from build123d import *

# Parameters (mm, degrees)
F0_R     = 25.118171
F0_R_2   = 20.499511
F1_DEPTH = 3
F0_R_3   = 15.56051
F2_DEPTH = 6
F0_R_4   = 10.077098
F3_DEPTH = 9
F0_R_5   = 4.284834
F4_DEPTH = 12
F0_R_6   = 1.253912
F5_DEPTH = 15
F6_DEPTH = 15
F7_DEPTH = 15


with BuildPart() as f1:
    # F0 (on Front) → F1 (new body)
    with BuildSketch(Plane.XZ):
        Circle(F0_R)
        Circle(F0_R_2, mode=Mode.SUBTRACT)
    extrude(amount=F1_DEPTH)

    # F0 (on Front) → F2 (join)
    with BuildSketch(Plane.XZ):
        Circle(F0_R_2)
        Circle(F0_R_3, mode=Mode.SUBTRACT)
    extrude(amount=F2_DEPTH)

    # F0 (on Front) → F3 (join)
    with BuildSketch(Plane.XZ):
        Circle(F0_R_3)
        Circle(F0_R_4, mode=Mode.SUBTRACT)
    extrude(amount=F3_DEPTH)

    # F0 (on Front) → F4 (join)
    with BuildSketch(Plane.XZ):
        Circle(F0_R_4)
        Circle(F0_R_5, mode=Mode.SUBTRACT)
    extrude(amount=F4_DEPTH)

    # F0 (on Front) → F5 (join)
    with BuildSketch(Plane.XZ):
        Circle(F0_R_5)
        Circle(F0_R_6, mode=Mode.SUBTRACT)
    extrude(amount=F5_DEPTH)

    # F0 (on Front) → F6 (join)
    with BuildSketch(Plane.XZ):
        Circle(F0_R_6)
    extrude(amount=F6_DEPTH)

    # F0 (on Front) → F7 (join)
    with BuildSketch(Plane.XZ):
        Circle(F0_R_6)
    extrude(amount=-F7_DEPTH)


solid = f1.part
For this review, take the finished solid that the model builds, in its own axes (mm). A direction names the side the tool comes from. Round coordinates to 2 decimals unless told otherwise and drop trailing zeros. Write each loop counter-clockwise with the first axis right and the second up, starting at its lowest first coordinate (ties: lowest second). Pieces come first, ordered by that corner, then holes. Notation, with made-up numbers: (-31, -8.75) -> (19, -8.75) arc R14 cw to (19, -4.75) -> close; hole circle Ø2 at (89.5, 66.25). An arc over 180 degrees is marked (long way). Use CSV: the item, a comma, the result in double quotes.
(1) Consider section A-A, the plane x = 0. Give the boundary of the cut face in (y, z).
Computed values:
outline,"(-15, -4.28) -> (-12, -4.28) -> (-12, -10.08) -> (-9, -10.08) -> (-9, -15.56) -> (-6, -15.56) -> (-6, -20.5) -> (-3, -20.5) -> (-3, -25.12) -> (0, -25.12) -> (0, -1.25) -> (15, -1.25) -> (15, 1.25) -> (0, 1.25) -> (0, 25.12) -> (-3, 25.12) -> (-3, 20.5) -> (-6, 20.5) -> (-6, 15.56) -> (-9, 15.56) -> (-9, 10.08) -> (-12, 10.08) -> (-12, 4.28) -> (-15, 4.28) -> close"
(2) Draft analysis for pull direction Z (two halves, no side actions). For faces 1 (the face through (-4.444, -4.479, -20.012)), 2 (the face through (3, -9, -10)), state which applies: +Z half, -Z half, draft (parallel to the pull), parting line (faces both ways), or undercut.
Computed values:
face 1,"parting line"
face 2,"draft"
(3) To check wall thickness, follow L1, parallel to Y at x = 7.5, z = -4.5; L2, parallel to Y at x = 18.5, z = -6; L3, parallel to X at y = -6.5, z = -6.5. State the ranges of each line that lie inside material, in increasing order. Write a range as [from, to].
Computed values:
L1,"[-12, 0]"
L2,"[-6, 0]"
L3,"[-14.14, 14.14]"
(4) For faces 3 (the face through (2, -12, -4)), 4 (the face through (-0.163, 7.395, 1.243)), 5 (the face through (0, -15, 0)), list the 3-axis set-ups (+Z, -Z, +X, -X, +Y, -Y) from which the entire face can be reached by the end or side of a thin tool; tool diameter is ignored.
Computed values:
face 3,"-Y"
face 4,"+Y"
face 5,"+Z, -Z, +X, -X, -Y"
(5) Consider section D-D, the plane z = 9. Give the boundary of the cut face in (x, y), plus the area to 3 significant figures.
Computed values:
outline,"(-23.45, -3) -> (-18.42, -3) -> (-18.42, -6) -> (-12.69, -6) -> (-12.69, -9) -> (-4.53, -9) -> (-4.53, -12) -> (4.53, -12) -> (4.53, -9) -> (12.69, -9) -> (12.69, -6) -> (18.42, -6) -> (18.42, -3) -> (23.45, -3) -> (23.45, 0) -> (-23.45, 0) -> close"
area,"355 mm²"
(6) Clearance check with flat-ended pins moving along their axes: P1, Ø2, axis at x = -16.5, y = -9.5, coming from the -Z side; P2, Ø5, axis at x = -16.5, z = -11.5, coming from the -Y side; P3, Ø1.5, axis at x = -13, y = -0.5, coming from the -Z side; P4, Ø4, axis at y = -9.5, z = 15, coming from the -X side. State where each tip first meets the part, or that it passes through.
Computed values:
P1,"through"
P2,"y = -6"
P3,"z = -21.93"
P4,"x = -8.45"
(7) Consider section C-C, the plane y = 11.25. Give the boundary of the cut face in (x, z).
Computed values:
outline,"circle Ø2.51 at (0, 0)"
(8) Consider section B-B, the plane z = 0. Give the boundary of the cut face in (x, y).
Computed values:
outline,"(-25.12, -3) -> (-20.5, -3) -> (-20.5, -6) -> (-15.56, -6) -> (-15.56, -9) -> (-10.08, -9) -> (-10.08, -12) -> (-4.28, -12) -> (-4.28, -15) -> (4.28, -15) -> (4.28, -12) -> (10.08, -12) -> (10.08, -9) -> (15.56, -9) -> (15.56, -6) -> (20.5, -6) -> (20.5, -3) -> (25.12, -3) -> (25.12, 0) -> (1.25, 0) -> (1.25, 15) -> (-1.25, 15) -> (-1.25, 0) -> (-25.12, 0) -> close"
